Read the model definition and answer for the solid it produces. Units are mm, in the model's axes. Face numbers are marked on the shaded views. A direction names the side the tool comes from. Coordinates: 2 decimals unless noted, no trailing zeros. Loops run counter-clockwise (first coordinate to the right, second up) from the corner with the lowest first, then second, coordinate; pieces in that order, holes last. Notation, with made-up numbers: M 9.5,44 L 18.5,44 A30 cw 18.5,66 Z; hole C 88,85 d11. An arc over 180 degrees is marked long. Use one line per item in the form item = value. Start each with the question number.
1. For a pull along Z with two mould halves and no side action, classify the marked faces 3, 4 and 5 as released by +Z, released by -Z, zero draft, split by the parting line, or undercut.
2. Flat-ended cylindrical pins translate along their axes: pin 1 (8 mm diameter, centred on y = -13, z = 44, fed in from +X); pin 2 (8 mm diameter, centred on x = -40, y = 22.5, fed in from -Z); pin 3 (2 mm diameter, centred on y = -24.5, z = 79.5, fed in from +X). Find the tip coordinate at first contact, or state that the pin passes through.
3. A tool of negligible diameter and unlimited length cuts with its end or side. For the marked faces 1 and 2, from which of +Z, -Z, +X, -X, +Y, -Y can it reach the whole face along a straight path? Write none if from no direction.
4. Find the intervals of material crossed by probe 1 along Z at (x, y) = (-50, 37); probe 2 along Y at (x, z) = (-57.5, 197); probe 3 along Y at (x, z) = (52.5, 289), in increasing order. Write a range as [from, to].
5. The part is cut by section D-D (x = -55). Give the vertices of the cut face in (y, z), plus the area to 3 significant figures.
6. The part is cut by section A-A (x = 0). Give the vertices of the cut face in (y, z).
7. The part is cut by section B-B (x = 45). Give the vertices of the cut face in (y, z).
from build123d import *

# Parameters (mm, degrees)
F0_W     = 127
F0_H     = 127
F0_R     = 25.4
F1_DEPTH = 25.4
F2_DEPTH = 355.6
F3_W     = 127
F3_H     = 127
F3_R     = 25.4
F4_DEPTH = 228.6
F5_R     = 12.7


with BuildPart() as f1:
    # F0 (on Top) → F1 (new body)
    with BuildSketch(Plane.XY):
        Rectangle(F0_W, F0_H)
        Circle(F0_R, mode=Mode.SUBTRACT)
    extrude(amount=F1_DEPTH)

    # F0 (on Top) → F2 (join)
    with BuildSketch(Plane.XY):
        Circle(F0_R)
    extrude(amount=F2_DEPTH)

    # F3 (on face) → F4 (join)
    with BuildSketch(Plane.XY.offset(355.6)):
        Rectangle(F3_W, F3_H)
        Circle(F3_R)
    extrude(amount=-F4_DEPTH)

    # F5
    f5_edges = [f1.edges().sort_by_distance(p)[0] for p in [
        (63.5, -63.5, 241.3),
        (63.5, 63.5, 241.3),
        (-63.5, -63.5, 241.3),
        (63.5, -63.5, 12.7),
        (63.5, 63.5, 12.7),
        (-63.5, -63.5, 12.7),
        (-63.5, 63.5, 241.3),
        (-63.5, 63.5, 12.7),
    ]]
    fillet(f5_edges, radius=F5_R)


solid = f1.part
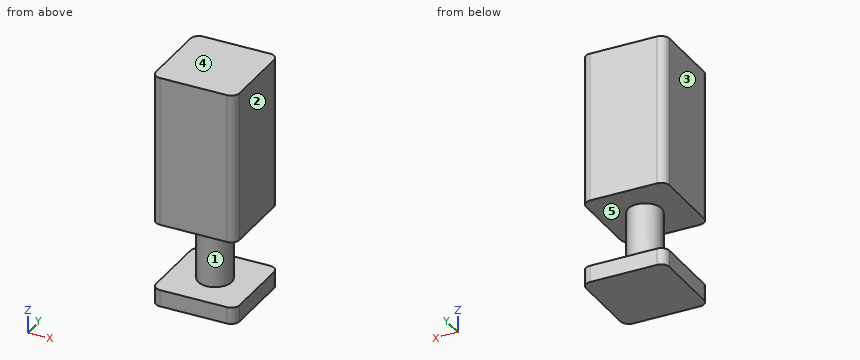
Computed values:
q1.face_3 = zero draft
q1.face_4 = released by +Z
q1.face_5 = undercut
q2.pin_1 = 23.75
q2.pin_2 = 0
q2.pin_3 = 9.64
q3.face_1 = none
q3.face_2 = +Z, -Z, +X, +Y, -Y
q4.probe_1 = [0, 25.4], [127, 355.6]
q4.probe_2 = [-61.59, 61.59]
q4.probe_3 = [-63.39, 63.39]
q5.outline = M -62.79,0 L 62.79,0 L 62.79,25.4 L -62.79,25.4 Z; M -62.79,127 L 62.79,127 L 62.79,355.6 L -62.79,355.6 Z
q5.area = 31,900 mm²
q6.outline = M -63.5,0 L 63.5,0 L 63.5,25.4 L 25.4,25.4 L 25.4,127 L 63.5,127 L 63.5,355.6 L -63.5,355.6 L -63.5,127 L -25.4,127 L -25.4,25.4 L -63.5,25.4 Z
q7.outline = M -63.5,0 L 63.5,0 L 63.5,25.4 L -63.5,25.4 Z; M -63.5,127 L 63.5,127 L 63.5,355.6 L -63.5,355.6 Z
